Geometry: final body of the model. Coordinates: model frame, mm. A direction names the side the tool comes from. Give positions to 0.01 mm unless a question says otherwise; leave off trailing zeros. One line per question, with ' | ' between items. Start each with the question number.
Item 1: Mould query, pull axis X, two halves, no side actions, for faces 1 (the flat face through (133, -15, 0)), 2 (the cylindrical face through (190.11, 28.21, 6.44)). Classes: released by +X, released by -X, zero draft, split by the parting line, or undercut.
Item 2: Set-up query: faces 3 (the cylindrical face through (2.213, -16.855, 7.193)), 4 (the cylindrical face through (-9.139, 14.334, 1.972)), 5 (the flat face through (93.247, 7.926, 6.439)). Return all of +Z, -Z, +X, -X, +Y, -Y with unobstructed straight access to the full face (end or side cutting, diameter ignored); none if empty.
Item 3: Material intervals for line 1 along X through (y, z) = (-2, 8.5); line 2 along Z through (x, y) = (-23, 11); line 3 along Y through (x, z) = (14, 11.5), sorted ascending. Write a range as [from, to].
Item 4: Pin query (flat end, axial travel): P1, Ø3.5, axis at x = 12.56, y = 3.36, coming from the +Z side; P2, Ø1.5, axis at x = 2.5, z = 10.5, coming from the +Y side; P3, Ø4, axis at x = 0, y = 22, coming from the -Z side. Return the tip coordinate at first contact, or that it passes through.
from build123d import *

# Parameters (mm, degrees)
SALIENTE_EXTRUIR1_DEPTH = 12.7
CORTAR_EXTRUIR20_DEPTH  = 62
CROQUIS12_R             = 26
CROQUIS12_R_2           = 17
CORTAR_EXTRUIR21_DEPTH  = 4
CROQUIS6_R              = 1.25
CORTAR_EXTRUIR22_DEPTH  = 29
CROQUIS13_R             = 1.5
CORTAR_EXTRUIR23_DEPTH  = 29
CROQUIS8_R              = 3
CORTAR_EXTRUIR27_DEPTH  = 64
CROQUIS5_R              = 36
CORTAR_EXTRUIR28_DEPTH  = 4
CROQUIS22_R             = 27
CORTAR_EXTRUIR32_DEPTH  = 1
CORTAR_EXTRUIR33_START  = -1
CROQUIS23_R             = 17
CORTAR_EXTRUIR33_DEPTH  = 1
CROQUIS24_R             = 9
CORTAR_EXTRUIR34_DEPTH  = 67
CROQUIS26_R             = 37
CROQUIS26_R_2           = 26.5
CORTAR_EXTRUIR38_DEPTH  = 9


with BuildPart() as part:
    # Croquis2 → Saliente-Extruir1 (new body)
    with BuildSketch(Plane.XY):
        with BuildLine():
            add(Edge.make_bspline(
                [(318.003849686, 21.000507192), (228.612845689, 50.579171404), (93.837740705, 69.713331037), (-40.897656903, 33.469788637), (-68.237071347, 4.559111896)],
                knots=[0, 0, 0, 0, 0.7074371, 1, 1, 1, 1], degree=3))
            Line((-68.237071347, 4.559111896), (-59.653213383, -5.20395025))
            add(Edge.make_bspline(
                [(-31, -25), (-39.39631193, -15.138516418), (-48.385558495, -7.834552383), (-59.653213383, -5.20395025)],
                knots=[0.5325633, 0.5325633, 0.5325633, 0.5325633, 1, 1, 1, 1], degree=3))
            add(Edge.make_bspline(
                [(0, -42), (-18.317933693, -37.788499598), (-31, -25)],
                knots=[0, 0, 0, 0.892929879, 0.892929879, 0.892929879], degree=2))
            add(Edge.make_bspline(
                [(0, -42), (34.804106533, -48.583870116), (140.601557422, -28.662967351), (242.066250638, 5.979270436), (318.003849686, -15.054295763)],
                knots=[0, 0, 0, 0, 0.322299538, 1, 1, 1, 1], degree=3))
            ThreePointArc((318.003849686, -15.054295763), (319.540823222, -15.003980459), (321.071215203, -14.853250005))
            ThreePointArc((321.071215203, -14.853250005), (322.775428516, -14.025460634), (323.64375194, -12.341538815))
            add(Edge.make_bspline(
                [(338, 6.2), (337.96483394, 6.165565228), (334.391730923, 4.926696382), (325.456575586, -0.138969503), (325.231234185, -2.170240746), (323.64375194, -12.341538815)],
                knots=[0.205943753, 0.205943753, 0.205943753, 0.205943753, 0.210383616, 0.534400108, 0.959977028, 0.959977028, 0.959977028, 0.959977028], degree=3))
            ThreePointArc((338, 6.2), (339.38638351, 10.840617369), (336.189590247, 14.479010095))
            Line((336.189590247, 14.479010095), (318.003849686, 21.000507192))
        make_face()
    extrude(amount=SALIENTE_EXTRUIR1_DEPTH)

    # Croquis15 → Cortar-Extruir20 (cut)
    with BuildSketch(Plane.XY.offset(12.7)):
        with BuildLine():
            Line((97.723501447, -12.756776492), (105.361190757, 30.558712033))
            ThreePointArc((105.361190757, 30.558712033), (107.138627567, 33.576200952), (110.459727005, 34.68742528))
            Line((110.459727005, 34.68742528), (185.414039032, 32.069963027))
            ThreePointArc((185.414039032, 32.069963027), (190.128162759, 28.12247669), (187.449594034, 22.587959504))
            Line((187.449594034, 22.587959504), (104.857592698, -18.110066768))
            ThreePointArc((104.857592698, -18.110066768), (99.646563775, -17.624284866), (97.723501447, -12.756776492))
        make_face()
        with BuildLine():
            Line((89.822655638, -11.494535825), (96.768582744, 27.897774295))
            ThreePointArc((96.768582744, 27.897774295), (95.058482028, 32.596237399), (90.134443263, 33.464478287))
            Line((90.134443263, 33.464478287), (52.546738431, 19.783672554))
            ThreePointArc((52.546738431, 19.783672554), (49.332800383, 15.953450339), (51.0429011, 11.254987235))
            Line((51.0429011, 11.254987235), (81.684678824, -14.456517153))
            ThreePointArc((81.684678824, -14.456517153), (86.608717589, -15.324758041), (89.822655638, -11.494535825))
        make_face()
        with BuildLine():
            Line((178.485600868, 8.76169092), (208.786453861, 25.718640542))
            ThreePointArc((208.786453861, 25.718640542), (210.340015249, 26.275882173), (211.990356529, 26.296974372))
            Line((211.990356529, 26.296974372), (242.009853595, 21.667000055))
            ThreePointArc((242.009853595, 21.667000055), (246.246230456, 16.846807749), (242.248805987, 11.826674245))
            Line((242.248805987, 11.826674245), (181.928455927, -0.50030106))
            ThreePointArc((181.928455927, -0.50030106), (176.240671419, 2.65632611), (178.485600868, 8.76169092))
        make_face()
    extrude(amount=-CORTAR_EXTRUIR20_DEPTH, mode=Mode.SUBTRACT)

    # Croquis12 → Cortar-Extruir21 (cut)
    with BuildSketch(Plane(origin=(0, 0, 0), x_dir=(-1, 0, 0), z_dir=(0, 0, -1))):
        Circle(CROQUIS12_R)
        Circle(CROQUIS12_R_2, mode=Mode.SUBTRACT)
    extrude(amount=-CORTAR_EXTRUIR21_DEPTH, mode=Mode.SUBTRACT)

    # Croquis6 → Cortar-Extruir22 (cut)
    with BuildSketch(Plane.XY.offset(12.7)):
        with Locations((0, 22)):
            Circle(CROQUIS6_R)
        with Locations((11, 19.052558883)):
            Circle(CROQUIS6_R)
        with Locations((19.052558883, 11)):
            Circle(CROQUIS6_R)
        with Locations((22, 0)):
            Circle(CROQUIS6_R)
        with Locations((19.052558883, -11)):
            Circle(CROQUIS6_R)
        with Locations((11, -19.052558883)):
            Circle(CROQUIS6_R)
        with Locations((0, -22)):
            Circle(CROQUIS6_R)
        with Locations((-11, -19.052558883)):
            Circle(CROQUIS6_R)
        with Locations((-19.052558883, -11)):
            Circle(CROQUIS6_R)
        with Locations((-22, 0)):
            Circle(CROQUIS6_R)
        with Locations((-19.052558883, 11)):
            Circle(CROQUIS6_R)
        with Locations((-11, 19.052558883)):
            Circle(CROQUIS6_R)
    extrude(amount=-CORTAR_EXTRUIR22_DEPTH, mode=Mode.SUBTRACT)

    # Croquis13 → Cortar-Extruir23 (cut)
    with BuildSketch(Plane(origin=(0, 0, 0), x_dir=(-1, 0, 0), z_dir=(0, 0, -1))):
        with Locations((12.557035742, -3.364647586)):
            Circle(CROQUIS13_R)
        with Locations((3.364647586, -12.557035742)):
            Circle(CROQUIS13_R)
        with Locations((-9.192388155, -9.192388155)):
            Circle(CROQUIS13_R)
        with Locations((9.192388155, 9.192388155)):
            Circle(CROQUIS13_R)
        with Locations((-12.557035742, 3.364647586)):
            Circle(CROQUIS13_R)
        with Locations((-3.364647586, 12.557035742)):
            Circle(CROQUIS13_R)
    extrude(amount=-CORTAR_EXTRUIR23_DEPTH, mode=Mode.SUBTRACT)

    # Croquis8 → Cortar-Extruir27 (cut)
    with BuildSketch(Plane.XY.offset(12.7)):
        with Locations((319.95126245, 5.58477006)):
            Circle(CROQUIS8_R)
    extrude(amount=-CORTAR_EXTRUIR27_DEPTH, mode=Mode.SUBTRACT)

    # Croquis5 → Cortar-Extruir28 (cut)
    with BuildSketch(Plane.XY.offset(12.7)):
        Circle(CROQUIS5_R)
    extrude(amount=-CORTAR_EXTRUIR28_DEPTH, mode=Mode.SUBTRACT)

    # Croquis22 → Cortar-Extruir32 (cut)
    with BuildSketch(Plane.XY.offset(8.7)):
        Circle(CROQUIS22_R)
    extrude(amount=-CORTAR_EXTRUIR32_DEPTH, mode=Mode.SUBTRACT)

    # Croquis23 → Cortar-Extruir33 (cut)
    with BuildSketch(Plane.XY.offset(7.7).offset(CORTAR_EXTRUIR33_START)):
        with Locations(Location((0, 0, 0), (0, 0, 180))):
            Circle(CROQUIS23_R)
    extrude(amount=CORTAR_EXTRUIR33_DEPTH, mode=Mode.SUBTRACT)

    # Croquis24 → Cortar-Extruir34 (cut)
    with BuildSketch(Plane(origin=(0, 0, 0), x_dir=(-1, 0, 0), z_dir=(0, 0, -1))):
        Circle(CROQUIS24_R)
    extrude(amount=-CORTAR_EXTRUIR34_DEPTH, mode=Mode.SUBTRACT)

    # Croquis26 → Cortar-Extruir38 (cut)
    with BuildSketch(Plane.XY.offset(12.7)):
        Circle(CROQUIS26_R)
        Circle(CROQUIS26_R_2, mode=Mode.SUBTRACT)
    extrude(amount=-CORTAR_EXTRUIR38_DEPTH, mode=Mode.SUBTRACT)


solid = part.part
Result sheet:
1) face 1: zero draft | face 2: undercut
2) face 3: +Z | face 4: -Z | face 5: +Z, -Z
3) line 1: x = [-62.47, -36.95], [36.95, 66.84], [91.5, 99.62], [137.55, 325.68] | line 2: z = [4, 7.7] | line 3: y = [-43.98, -34.25], [34.25, 45.66]
4) P1: stops at z = 6.7 | P2: stops at y = 43.13 | P3: stops at z = 4
